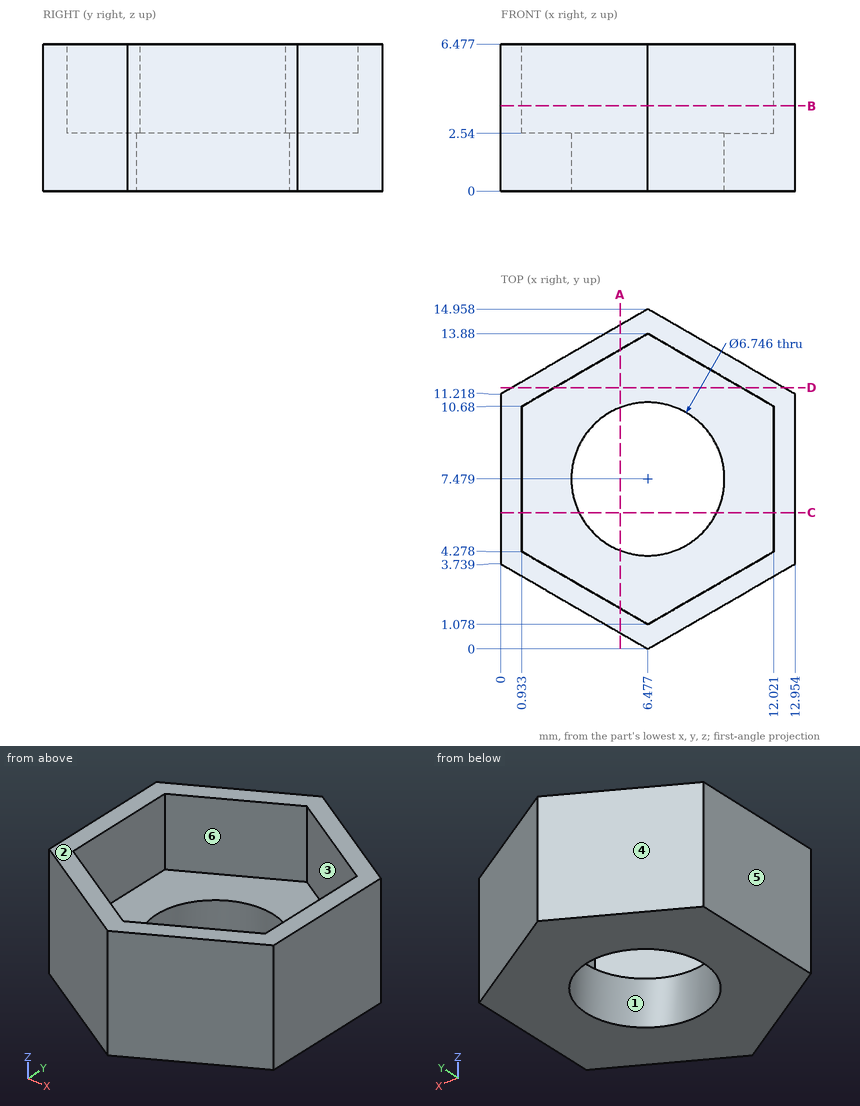
Source: three-view drawing plus pictorial views. Frame: mm from the lowest corner of the part. A direction names the side the tool comes from. Coordinates: 2 decimals unless noted, no trailing zeros. Order: outer loops, then holes, each group sorted by start corner. A loop starts at its lowest first (then second) coordinate and runs counter-clockwise, first axis right, second up. Notation, with made-up numbers: M 81,81 L 115,81 A24 cw 115,120 Z; hole C -12,30.5 d6. An arc over 180 degrees is marked long. Answer in a Markdown table with one row per item.
(1) Section query D-D, the plane y = 11.5. Output: boundary loops of the cut face in (x, z) (1 decimal).
Numbers:
| item | result |
|---|---|
| outline | M 0.5,0 L 12.5,0 L 12.5,6.5 L 10.6,6.5 L 10.6,2.5 L 2.4,2.5 L 2.4,6.5 L 0.5,6.5 Z |
(2) Access query for the marked faces 5 and 6. Directions: +Z, -Z, +X, -X, +Y, -Y. A direction counts if a zero-diameter tool reaches every point of the face in a straight line with its end or side. Return the directions, or none.
Numbers:
| item | result |
|---|---|
| face 5 | +Z, -Z, -X, +Y, -Y |
| face 6 | +Z |
(3) Contact query for flat-ended pins moving along their axis: pin 1 Ø3.5 at (x, y) = (8.5, 8) entering from +Z; pin 2 Ø2 at (x, z) = (9.5, 2) entering from -Y. Output: stop coordinate, or through.
Numbers:
| item | result |
|---|---|
| pin 1 | stops at z = 2.54 |
| pin 2 | stops at y = 1.17 |
(4) Section query B-B, the plane z = 3.75. Output: boundary loops of the cut face in (x, y) (1 decimal).
Numbers:
| item | result |
|---|---|
| outline | M 0,3.7 L 6.5,0 L 13,3.7 L 13,11.2 L 6.5,15 L 0,11.2 Z; hole M 0.9,4.3 L 6.5,1.1 L 12,4.3 L 12,10.7 L 6.5,13.9 L 0.9,10.7 Z |
(5) Section query A-A, the plane x = 5.25. Output: boundary loops of the cut face in (y, z).
Numbers:
| item | result |
|---|---|
| outline | M 0.71,0 L 4.34,0 L 4.34,2.54 L 1.79,2.54 L 1.79,6.48 L 0.71,6.48 Z; M 10.62,0 L 14.25,0 L 14.25,6.48 L 13.17,6.48 L 13.17,2.54 L 10.62,2.54 Z |
(6) Section query C-C, the plane y = 6. Output: boundary loops of the cut face in (x, z) (1 decimal).
Numbers:
| item | result |
|---|---|
| outline | M 0,0 L 3.4,0 L 3.4,2.5 L 0.9,2.5 L 0.9,6.5 L 0,6.5 Z; M 9.5,0 L 13,0 L 13,6.5 L 12,6.5 L 12,2.5 L 9.5,2.5 Z |
(7) Material intervals for line 1 (X direction, y = 7.75, z = 3.75) (1 decimal); line 2 (Y direction, x = 7.75, z = 0.75) (1 decimal); line 3 (Y direction, x = 7.5, z = 0.5) (1 decimal), sorted ascending. Write a range as [from, to].
Numbers:
| item | result |
|---|---|
| line 1 | x = [0, 0.9], [12, 13] |
| line 2 | y = [0.7, 4.4], [10.6, 14.2] |
| line 3 | y = [0.6, 4.3], [10.7, 14.4] |
(8) Draft query along Y for the marked faces 1, 2, 3 and 4. Return one class per face: pulls with the +Y half, pulls with the -Y half, needs draft (parallel to the pull), parting line crosses it, or undercut.
Numbers:
| item | result |
|---|---|
| face 1 | undercut |
| face 2 | needs draft |
| face 3 | undercut |
| face 4 | pulls with the +Y half |
